CAD build for the part. Positions are in the model's coordinates, mm. A direction names the side the tool comes from. Round coordinates to 2 decimals unless told otherwise and drop trailing zeros. Order: outer loops, then holes, each group sorted by start corner. A loop starts at its lowest first (then second) coordinate and runs counter-clockwise, first axis right, second up. Notation, with made-up numbers: M 5.25,-6.75 L 25.25,-6.75 A21 cw 25.25,3.25 Z; hole C -9.75,46.25 d10. An arc over 180 degrees is marked long. Answer as a JSON object with one key per item and string values.
```python
from build123d import *

# Parameters (mm, degrees)
CROQUIS1_R                 = 33
SALIENTE_EXTRUIR1_DEPTH    = 15
SALIENTE_EXTRUIR2_DEPTH    = 15
SALIENTE_EXTRUIR3_DEPTH    = 50
CROQUIS4_R                 = 33
SALIENTE_EXTRUIR4_DEPTH    = 60
CROQUIS5_R                 = 27.5
CORTAR_EXTRUIR1_DEPTH      = 40
CROQUIS6_R                 = 27.5
CORTAR_EXTRUIR2_DEPTH      = 75
CROQUIS7_R                 = 1
CORTAR_EXTRUIR3_DEPTH      = 61
CORTAR_EXTRUIR3_DEPTH_BACK = 61


with BuildPart() as part:
    # Croquis1 → Saliente-Extruir1 (new body, symmetric)
    with BuildSketch(Plane.XY):
        Circle(CROQUIS1_R)
    extrude(amount=SALIENTE_EXTRUIR1_DEPTH, both=True)

    # Croquis2 → Saliente-Extruir2 (add, symmetric)
    with BuildSketch(Plane.XY):
        with BuildLine():
            Line((-4.961389384, 39.691115069), (-4.093146241, 32.745169932))
            ThreePointArc((-4.093146241, 32.745169932), (-28.578838325, 16.5), (-30.404722133, -12.827816339))
            Line((-30.404722133, -12.827816339), (-36.854208646, -15.54886829))
            ThreePointArc((-36.854208646, -15.54886829), (-34.641016151, 20), (-4.961389384, 39.691115069))
        make_face()
        with BuildLine():
            Line((4.961389384, 39.691115069), (4.093146241, 32.745169932))
            ThreePointArc((4.093146241, 32.745169932), (28.578838325, 16.5), (30.404722133, -12.827816339))
            Line((30.404722133, -12.827816339), (36.854208646, -15.54886829))
            ThreePointArc((36.854208646, -15.54886829), (34.641016151, 20), (4.961389384, 39.691115069))
        make_face()
        with BuildLine():
            Line((31.892819262, -24.142246779), (26.311575891, -19.917353592))
            ThreePointArc((26.311575891, -19.917353592), (0, -33), (-26.311575891, -19.917353592))
            Line((-26.311575891, -19.917353592), (-31.892819262, -24.142246779))
            ThreePointArc((-31.892819262, -24.142246779), (0, -40), (31.892819262, -24.142246779))
        make_face()
    extrude(amount=SALIENTE_EXTRUIR2_DEPTH, both=True)

    # Croquis3 → Saliente-Extruir3 (add, symmetric)
    with BuildSketch(Plane.XY):
        with BuildLine():
            Line((-4.341215711, 34.729725685), (-4.961389384, 39.691115069))
            ThreePointArc((-4.961389384, 39.691115069), (-34.641016151, 20), (-36.854208646, -15.54886829))
            Line((-36.854208646, -15.54886829), (-32.247432565, -13.605259754))
            ThreePointArc((-32.247432565, -13.605259754), (-30.310889132, 17.5), (-4.341215711, 34.729725685))
        make_face()
        with BuildLine():
            Line((4.341215711, 34.729725685), (4.961389384, 39.691115069))
            ThreePointArc((4.961389384, 39.691115069), (34.641016151, 20), (36.854208646, -15.54886829))
            Line((36.854208646, -15.54886829), (32.247432565, -13.605259754))
            ThreePointArc((32.247432565, -13.605259754), (30.310889132, 17.5), (4.341215711, 34.729725685))
        make_face()
        with BuildLine():
            Line((31.892819262, -24.142246779), (27.906216854, -21.124465931))
            ThreePointArc((27.906216854, -21.124465931), (0, -35), (-27.906216854, -21.124465931))
            Line((-27.906216854, -21.124465931), (-31.892819262, -24.142246779))
            ThreePointArc((-31.892819262, -24.142246779), (0, -40), (31.892819262, -24.142246779))
        make_face()
    extrude(amount=SALIENTE_EXTRUIR3_DEPTH, both=True)

    # Croquis4 → Saliente-Extruir4 (add, symmetric)
    with BuildSketch(Plane.XY):
        Circle(CROQUIS4_R)
    extrude(amount=SALIENTE_EXTRUIR4_DEPTH, both=True)

    # Croquis5 → Cortar-Extruir1 (cut)
    with BuildSketch(Plane.XY.offset(60)):
        Circle(CROQUIS5_R)
    extrude(amount=-CORTAR_EXTRUIR1_DEPTH, mode=Mode.SUBTRACT)

    # Croquis6 → Cortar-Extruir2 (cut)
    with BuildSketch(Plane(origin=(0, 0, -60), x_dir=(-1, 0, 0), z_dir=(0, 0, -1))):
        Circle(CROQUIS6_R)
    extrude(amount=-CORTAR_EXTRUIR2_DEPTH, mode=Mode.SUBTRACT)

    # Croquis7 → Cortar-Extruir3 (cut, two sides)
    with BuildSketch(Plane.XY) as cortar_extruir3_sk:
        with Locations((5, 5)):
            Circle(CROQUIS7_R)
        with Locations((-5, 5)):
            Circle(CROQUIS7_R)
        with Locations((-5, -5)):
            Circle(CROQUIS7_R)
        with Locations((5, -5)):
            Circle(CROQUIS7_R)
    extrude(amount=CORTAR_EXTRUIR3_DEPTH, mode=Mode.SUBTRACT)
    extrude(cortar_extruir3_sk.sketch, amount=-CORTAR_EXTRUIR3_DEPTH_BACK, mode=Mode.SUBTRACT)


solid = part.part
```
Item 1: Two-plate mould, pull along Y, no slides. Class faces 5 (the cylindrical face through (-34.897, 19.551, -0.7)), 6 (the cylindrical face through (-30.534, 17.107, 32.255)), 7 (the flat face through (-12, 25, 60)), 8 (the flat face through (-30, 16, -15)): released by +Y, released by -Y, zero draft, split by the parting line, or undercut.
Worked answers:
{"face 5": "split by the parting line", "face 6": "undercut", "face 7": "zero draft", "face 8": "undercut"}
Item 2: Saw through at B-B on y = 0. List the corners of the cut face in (x, z), and give its area (4 significant figures).
Worked answers:
{"outline": "M -40,-50 L -35,-50 L -35,-15 L -33,-15 L -33,-60 L -27.5,-60 L -27.5,15 L 27.5,15 L 27.5,-60 L 33,-60 L 33,-15 L 35,-15 L 35,-50 L 40,-50 L 40,50 L 35,50 L 35,15 L 33,15 L 33,60 L 27.5,60 L 27.5,20 L -27.5,20 L -27.5,60 L -33,60 L -33,15 L -35,15 L -35,50 L -40,50 Z", "area": "2,715 mm2"}
Item 3: Saw through at C-C on z = 8. List the corners of the cut face in (x, y), and give its area (3 significant figures).
Worked answers:
{"outline": "M -36.85,-15.55 L -30.4,-12.83 A33 ccw -26.31,-19.92 L -31.89,-24.14 A40 ccw 31.89,-24.14 L 26.31,-19.92 A33 ccw 30.4,-12.83 L 36.85,-15.55 A40 ccw 4.96,39.69 L 4.09,32.75 A33 ccw -4.09,32.75 L -4.96,39.69 A40 ccw Z; hole C 0,0 d55", "area": "2,460 mm2"}
Item 4: Saw through at A-A on z = 48.5. List the corners of the cut face in (x, y), and give its area (3 significant figures).
Worked answers:
{"outline": "M -36.85,-15.55 L -32.25,-13.61 A35 cw -4.34,34.73 L -4.96,39.69 A40 ccw Z; C 0,0 d66; M -31.89,-24.14 A40 ccw 31.89,-24.14 L 27.91,-21.12 A35 cw -27.91,-21.12 Z; M 4.34,34.73 A35 cw 32.25,-13.61 L 36.85,-15.55 A40 ccw 4.96,39.69 Z; hole C 0,0 d55", "area": "2,080 mm2"}
Item 5: Drop flat-ended pins along their axis: pin 1 Ø8 at (x, y) = (-2.5, 16) entering from +Z; pin 2 Ø10 at (y, z) = (-31.5, 14.5) entering from -X; pin 3 Ø1 at (y, z) = (-22.5, 14) entering from +X; pin 4 Ø15.5 at (x, y) = (-19.5, 15) entering from +Z. Give the stop position or say it passes through.
Worked answers:
{"pin 1": "stops at z = 20", "pin 2": "stops at x = -29.96", "pin 3": "stops at x = 30.38", "pin 4": "stops at z = 60"}
Item 6: Wall check: line 1 along Y through (x, z) = (-29, 40); line 2 along Y through (x, z) = (0, -12); line 3 along X through (y, z) = (9, -42.5). Give the ranges that are in metal, low to high. Write a range as [from, to].
Worked answers:
{"line 1": "y = [-27.55, -21.95], [-15.75, 15.75], [19.6, 27.55]", "line 2": "y = [-40, -27.5], [27.5, 33]", "line 3": "x = [-38.97, -33.82], [-31.75, -25.99], [25.99, 31.75], [33.82, 38.97]"}
Item 7: 3-axis set-ups, long thin cutter, end or side, ignore diameter. For faces 1 (the flat face through (0, -36, -50)), 2 (the flat face through (0, -36, 50)), 3 (the cylindrical face through (-5.961, -26.846, 40.28)), 4 (the flat face through (29, 18, -15)): which of +Z, -Z, +X, -X, +Y, -Y reach the whole face in a straight line?
Worked answers:
{"face 1": "-Z, -Y", "face 2": "+Z, -Y", "face 3": "+Z", "face 4": "-Z"}
Item 8: Saw through at D-D on x = -24.5. List the corners of the cut face in (y, z) (3 decimals).
Worked answers:
{"outline": "M -31.619,-50 L -24.995,-50 L -24.995,-15 L -22.108,-15 L -22.108,-60 L -12.49,-60 L -12.49,15 L 12.49,15 L 12.49,-60 L 22.108,-60 L 22.108,-15 L 24.995,-15 L 24.995,-50 L 31.619,-50 L 31.619,50 L 24.995,50 L 24.995,15 L 22.108,15 L 22.108,60 L 12.49,60 L 12.49,20 L -12.49,20 L -12.49,60 L -22.108,60 L -22.108,15 L -24.995,15 L -24.995,50 L -31.619,50 Z"}
